Could you check a few things on this model? Use its own coordinates, in mm. A direction names the side the tool comes from. Round coordinates to 2 decimals unless told otherwise and drop trailing zeros. Write each loop counter-clockwise with the first axis right and the second up, starting at its lowest first coordinate (ties: lowest second). Pieces come first, ordered by that corner, then holes. Notation, with made-up numbers: (21.25, 31.5) -> (62.25, 31.5) arc R26 ccw to (62.25, 55.5) -> close; hole circle Ø1 at (-13.5, 55.5). An arc over 180 degrees is marked (long way). Return JSON: item names as keys, results as strings.
from build123d import *

# Parameters (mm, degrees)
BOSS_EXTRUDE1_DEPTH = 8
SKETCH3_R           = 6
SKETCH3_R_2         = 4
SKETCH3_R_3         = 9
CUT_EXTRUDE1_DEPTH  = 34
SKETCH5_R           = 6
BOSS_EXTRUDE2_DEPTH = 6
SKETCH6_R           = 4
BOSS_EXTRUDE3_DEPTH = 6


with BuildPart() as part:
    # Sketch2 → Boss-Extrude1 (new body)
    with BuildSketch(Plane(origin=(0, 0, 0), x_dir=(1, 0, 0), z_dir=(0, 1, 0))):
        with BuildLine():
            Line((14.773677032, 0), (74.248108018, 0))
            ThreePointArc((74.248108018, 0), (86.100368105, -10.12278642), (77.956311951, -23.412678196))
            Line((77.956311951, -23.412678196), (-3.116637066, -49.754876163))
            ThreePointArc((-3.116637066, -49.754876163), (-12.387146898, -49.754876163), (-19.887146898, -44.305807203))
            Line((-19.887146898, -44.305807203), (-62.224027937, 13.965910429))
            ThreePointArc((-62.224027937, 13.965910429), (-61.969059674, 23.702755576), (-52.497998837, 25.976556108))
            Line((-52.497998837, 25.976556108), (-2.309261977, 3.631090779))
            ThreePointArc((-2.309261977, 3.631090779), (6.041386017, 0.917800769), (14.773677032, 0))
        make_face()
    extrude(amount=BOSS_EXTRUDE1_DEPTH)

    # Sketch3 → Cut-Extrude1 (cut)
    with BuildSketch(Plane(origin=(0, 8, 0), x_dir=(1, 0, 0), z_dir=(0, 1, 0))):
        with Locations((74.248108018, -12)):
            Circle(SKETCH3_R)
        with Locations((-55.751891982, 18.668192447)):
            Circle(SKETCH3_R_2)
        with Locations((-7.751891982, -35.489028418)):
            Circle(SKETCH3_R_3)
    extrude(amount=-CUT_EXTRUDE1_DEPTH, mode=Mode.SUBTRACT)

    # Sketch5 → Boss-Extrude2 (add)
    with BuildSketch(Plane(origin=(14.894305626, 0, -4.83945326), x_dir=(-0.309016994, 0, -0.951056516), z_dir=(0.951056516, 0, -0.309016994))):
        with BuildLine():
            Line((-46.356605373, 8), (-46.356605373, 48))
            ThreePointArc((-46.356605373, 48), (-34.62942849, 60.519891788), (-22.367996489, 48.522739904))
            Line((-22.367996489, 48.522739904), (-13.754622225, 8))
            Line((-13.754622225, 8), (-46.356605373, 8))
        make_face()
        with Locations((-34.367996489, 48.522739904)):
            Circle(SKETCH5_R, mode=Mode.SUBTRACT)
    extrude(amount=-BOSS_EXTRUDE2_DEPTH)

    # Sketch6 → Boss-Extrude3 (add)
    with BuildSketch(Plane(origin=(-5.786875521, 0, -7.964950844), x_dir=(0.809016994, 0, -0.587785252), z_dir=(0.587785252, 0, 0.809016994))):
        with BuildLine():
            Line((-42.131339875, 8), (-42.131339875, 46))
            Line((-42.131339875, 46), (-42.131339875, 48))
            ThreePointArc((-42.131339875, 48), (-35.244724682, 55.92214455), (-26.441246307, 50.205098847))
            Line((-26.441246307, 50.205098847), (-14.339128957, 8))
            Line((-14.339128957, 8), (-42.131339875, 8))
        make_face()
        with Locations((-34.131339875, 48)):
            Circle(SKETCH6_R, mode=Mode.SUBTRACT)
    extrude(amount=BOSS_EXTRUDE3_DEPTH)


solid = part.part
1) I want a section at C-C, the plane z = -8. Please give me the cut outline in (x, y).
Return value:
{"outline": "(-57.89, 0) -> (-12.12, 0) -> (-12.12, 8) -> (-57.89, 8) -> close"}
2) I want a section at B-B, the plane x = 3. Please give me the cut outline in (y, z), and give its area (3 significant figures).
Return value:
{"outline": "(0, -1.68) -> (8, -1.68) -> (8, 47.77) -> (0, 47.77) -> close", "area": "396 mm²"}
3) Will these pins go through, and if not, where does the flat tip stop? pin 1 Ø15.5 at (x, z) = (74.25, 12) entering from +Y; pin 2 Ø7 at (x, z) = (-55.75, -18.67) entering from -Y; pin 3 Ø12 at (y, z) = (22, 36) entering from +X; pin 4 Ø2.5 at (x, y) = (53.5, 4) entering from -Z.
Return value:
{"pin 1": "y = 8", "pin 2": "through", "pin 3": "x = 29.22", "pin 4": "z = 0"}
4) For faces 1 (the face through (25.233, 28.793, 26.98)), 2 (the face through (44, 4, 0)), 3 (the face through (19.527, 28.793, 28.834)), 4 (the face through (17.68, 28.55, 13.31)), which set-ups out of +Z, -Z, +X, -X, +Y, -Y let a thin tool reach every point of the face, with its end or its side?
Return value:
{"face 1": "-Z, +X, +Y", "face 2": "-Z, +X, +Y, -Y", "face 3": "+Z, +Y", "face 4": "-Z, +Y"}
5) If I drill on probe 1 along Y at (x, z) = (-30, 1); probe 2 along X at (y, z) = (53, 19.5); probe 3 along X at (y, z) = (17, 17), over which ranges is the centre line in solid material (lowest first)? Write a range as [from, to].
Return value:
{"probe 1": "[0, 8]", "probe 2": "[-35.74, -33.38], [16.49, 22.8]", "probe 3": "[-39.73, -29.94], [15.68, 21.99]"}
6) I want a section at A-A, the plane y = 45.5. Please give me the cut outline in (x, z).
Return value:
{"outline": "(-39.87, 16.8) -> (-35.93, 13.93) -> (-32.4, 18.79) -> (-36.35, 21.65) -> close; (-30.87, 10.26) -> (-26.09, 6.78) -> (-22.56, 11.64) -> (-27.35, 15.12) -> close; (15.9, 17.68) -> (21.61, 15.82) -> (23.91, 22.92) -> (18.21, 24.77) -> close; (21.41, 34.63) -> (27.12, 32.78) -> (29.22, 39.25) -> (23.51, 41.1) -> close"}
7) Thinking about a two-plate mould opening in X: for faces 5 (the face through (-27.444, 27.003, 15.186)), 6 (the face through (-53.906, 4.056, -15.12)), 7 (the face through (-20.613, 29.398, 6.463)), 8 (the face through (-32.7, 55.9, 15.2)), which applies, pulls with the +X half, pulls with the -X half, needs draft (parallel to the pull), parting line crosses it, or undercut?
Return value:
{"face 5": "undercut", "face 6": "undercut", "face 7": "pulls with the +X half", "face 8": "parting line crosses it"}
